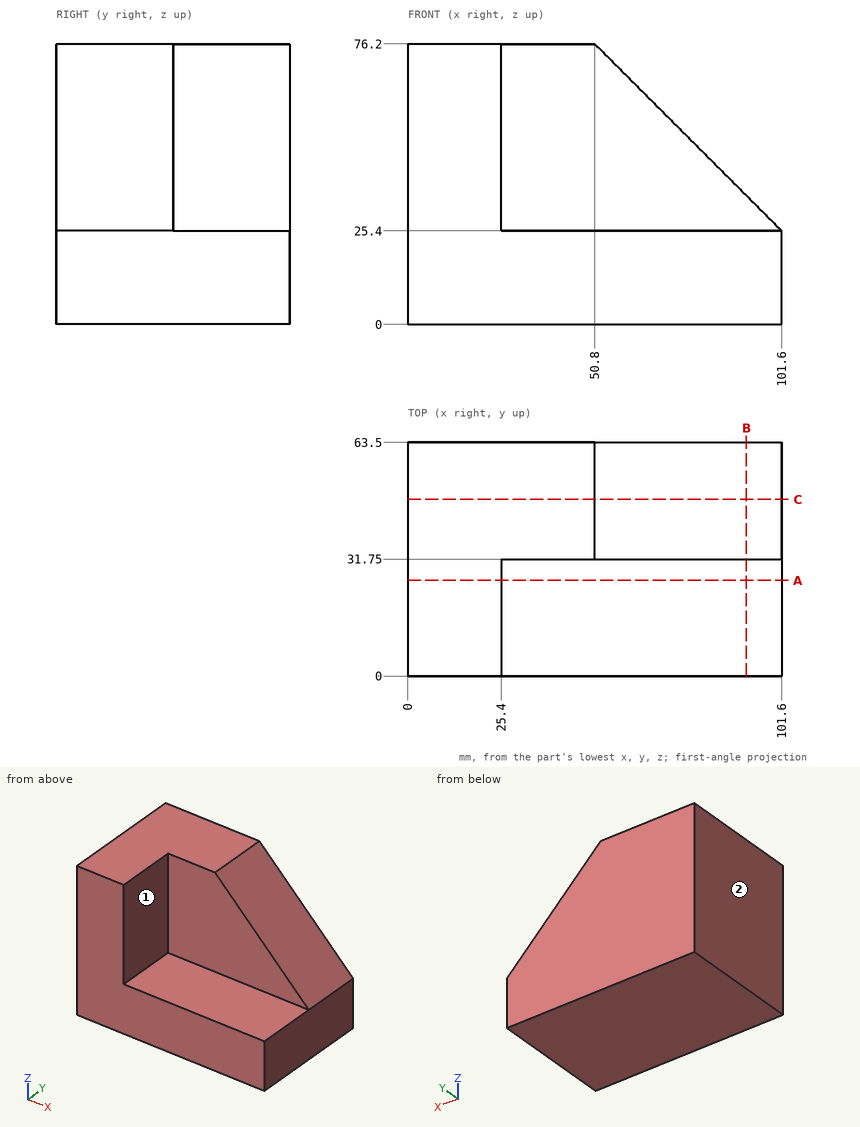
Job drawing, mm, ordinate dimensions from the low corner. One solid piece. A direction names the side the tool comes from. Give positions to 0.01 mm unless a question says otherwise; leave off trailing zeros. Loops run counter-clockwise (first coordinate to the right, second up) from the corner with the lowest first, then second, coordinate; pieces in that order, holes last. Notation, with made-up numbers: (4.25, -6) -> (12.25, -6) arc R8 cw to (12.25, -1) -> close; hole circle Ø2 at (66, -17). An arc over 180 degrees is marked (long way). Write each question's results on one line, items separated by ' | '.
(1) Probe line 1 along X through (y, z) = (14.5, 29.5); line 2 along Y through (x, z) = (49.5, 57). List the from-to ranges inside material, lowest first.
Geometry results:
line 1: x = 0 to 25.4 | line 2: y = 31.75 to 63.5
(2) Flat gauge pins, fed straight in: pin 1 Ø6 at (x, z) = (71.5, 41) entering from -Y; pin 2 Ø9.5 at (x, y) = (54.5, 21) entering from +Z. Where does each tip first touch, or does it go through?
Geometry results:
pin 1: stops at y = 31.75 | pin 2: stops at z = 25.4
(3) Cut at C-C on y = 48. List the corners of the cut face in (x, z), and give its area (3 significant figures).
Geometry results:
outline: (0, 0) -> (101.6, 0) -> (101.6, 25.4) -> (50.8, 76.2) -> (0, 76.2) -> close | area: 6,450 mm²
(4) Tool access for the marked faces 1 and 2: list every direction of +Z, -Z, +X, -X, +Y, -Y with a clear straight run to the whole face (end or side of a thin tool).
Geometry results:
face 1: +Z, +X, -Y | face 2: +Z, -Z, -X, +Y, -Y
(5) Cut at B-B on x = 92. List the corners of the cut face in (y, z), and give its area (3 significant figures).
Geometry results:
outline: (0, 0) -> (63.5, 0) -> (63.5, 35) -> (31.75, 35) -> (31.75, 25.4) -> (0, 25.4) -> close | area: 1,920 mm²
(6) Cut at A-A on y = 26. List the corners of the cut face in (x, z).
Geometry results:
outline: (0, 0) -> (101.6, 0) -> (101.6, 25.4) -> (25.4, 25.4) -> (25.4, 76.2) -> (0, 76.2) -> close
